```python
from build123d import *

# Parameters (mm, degrees)
EXTRUDE_1_DEPTH      = 6
SKETCH_2_W           = 10
SKETCH_2_H           = 5
CUT_EXTRUDE_1_DEPTH  = 31.822070015
SKETCH_3_R           = 1.5
CUT_EXTRUDE_2_DEPTH  = 39.013155617
SKETCH_4_W           = 20
SKETCH_4_H           = 34
CUT_EXTRUDE_3_DEPTH  = 2
SKETCH_5_R           = 1.25
CUT_EXTRUDE_4_DEPTH  = 31.495901364
FILLET_2_R           = 1.5
SKETCH_9_W           = 1.5
SKETCH_9_H           = 35
CUT_EXTRUDE_10_DEPTH = 31.822070015
SKETCH_10_W          = 2
SKETCH_10_H          = 6
EXTRUDE_2_DEPTH      = 6
SKETCH_11_R          = 1.25
CUT_EXTRUDE_11_DEPTH = 30.618406439


with BuildPart() as part:
    # 草图1 → 凸台-拉伸1 (new body)
    with BuildSketch(Plane.XY):
        Polygon((-25, -17), (-25, 17), (-22, 17), (-22, 11), (-12, 11), (-12, 17), (12, 17), (12, 11), (22, 11), (22, 17), (25, 17), (25, -17), (22, -17), (22, -11), (12, -11), (12, -17), (-12, -17), (-12, -11), (-22, -11), (-22, -17), align=None)
    extrude(amount=EXTRUDE_1_DEPTH)

    # 草图2 → 切除-拉伸1 (cut, through all)
    with BuildSketch(Plane.XY.offset(6)):
        with Locations((-16, 5)):
            Rectangle(SKETCH_2_W, SKETCH_2_H)
        with Locations((-16, -5)):
            Rectangle(SKETCH_2_W, SKETCH_2_H)
        with Locations((16, -5)):
            Rectangle(SKETCH_2_W, SKETCH_2_H)
        with Locations((16, 5)):
            Rectangle(SKETCH_2_W, SKETCH_2_H)
    extrude(amount=-CUT_EXTRUDE_1_DEPTH, mode=Mode.SUBTRACT)

    # 草图3 → 切除-拉伸2 (cut, through all)
    with BuildSketch(Plane.XZ.offset(11)):
        with Locations(Location((-16, 3, 0), (0, 0, 270))):
            Circle(SKETCH_3_R)
        with Locations(Location((16, 3, 0), (0, 0, 270))):
            Circle(SKETCH_3_R)
    extrude(amount=-CUT_EXTRUDE_2_DEPTH, mode=Mode.SUBTRACT)

    # 草图4 → 切除-拉伸3 (cut)
    with BuildSketch(Plane.XY.offset(6)):
        Rectangle(SKETCH_4_W, SKETCH_4_H)
    extrude(amount=-CUT_EXTRUDE_3_DEPTH, mode=Mode.SUBTRACT)

    # 草图5 → 切除-拉伸4 (cut, through all)
    with BuildSketch(Plane.XY.offset(4)):
        with Locations((-6, 6)):
            Circle(SKETCH_5_R)
        with Locations((6, 6)):
            Circle(SKETCH_5_R)
        with Locations((-6, -6)):
            Circle(SKETCH_5_R)
        with Locations((6, -6)):
            Circle(SKETCH_5_R)
    extrude(amount=-CUT_EXTRUDE_4_DEPTH, mode=Mode.SUBTRACT)

    # 圆角2
    fillet_2_edges = [part.edges().sort_by_distance(p)[0] for p in [
        (-11, 7.5, 3),
        (-11, 2.5, 3),
        (-21, 2.5, 3),
        (-21, 7.5, 3),
        (-21, -7.5, 3),
        (-21, -2.5, 3),
        (-11, -2.5, 3),
        (-11, -7.5, 3),
        (21, -2.5, 3),
        (21, -7.5, 3),
        (11, -7.5, 3),
        (11, -2.5, 3),
        (21, 7.5, 3),
        (21, 2.5, 3),
        (11, 2.5, 3),
        (11, 7.5, 3),
    ]]
    fillet(fillet_2_edges, radius=FILLET_2_R)

    # 草图9 → 切除-拉伸10 (cut, through all)
    with BuildSketch(Plane.XY.offset(6)):
        with Locations((-24.25, -0.5)):
            Rectangle(SKETCH_9_W, SKETCH_9_H)
        with Locations((24.25, -0.5)):
            Rectangle(SKETCH_9_W, SKETCH_9_H)
    extrude(amount=-CUT_EXTRUDE_10_DEPTH, mode=Mode.SUBTRACT)

    # 草图10 → 凸台-拉伸2 (add)
    with BuildSketch(Plane.XY.offset(6)):
        with Locations((-21, 14)):
            Rectangle(SKETCH_10_W, SKETCH_10_H)
        with Locations((21, 14)):
            Rectangle(SKETCH_10_W, SKETCH_10_H)
        with Locations((21, -14)):
            Rectangle(SKETCH_10_W, SKETCH_10_H)
        with Locations((-21, -14)):
            Rectangle(SKETCH_10_W, SKETCH_10_H)
    extrude(amount=-EXTRUDE_2_DEPTH)

    # 草图11 → 切除-拉伸11 (cut, through all)
    with BuildSketch(Plane.XY.offset(6)):
        with Locations((-19.2, 11.8)):
            Circle(SKETCH_11_R)
        with Locations((-12.8, 11.8)):
            Circle(SKETCH_11_R)
        with Locations((12.8, 11.8)):
            Circle(SKETCH_11_R)
        with Locations((19.2, 11.8)):
            Circle(SKETCH_11_R)
        with Locations((19.2, -11.8)):
            Circle(SKETCH_11_R)
        with Locations((12.8, -11.8)):
            Circle(SKETCH_11_R)
        with Locations((-12.8, -11.8)):
            Circle(SKETCH_11_R)
        with Locations((-19.2, -11.8)):
            Circle(SKETCH_11_R)
    extrude(amount=-CUT_EXTRUDE_11_DEPTH, mode=Mode.SUBTRACT)


solid = part.part
```
Part model, mm, in its own coordinate system. A direction names the side the tool comes from. Give positions to 0.01 mm unless a question says otherwise; leave off trailing zeros. Order: outer loops, then holes, each group sorted by start corner. A loop starts at its lowest first (then second) coordinate and runs counter-clockwise, first axis right, second up. Notation, with made-up numbers: M -26,66.5 L 4,66.5 A36 cw 4,105.5 Z; hole C 8.5,0 d10. An arc over 180 degrees is marked long. Use a Markdown table: item, result. Add a question column.
(1) Saw through at C-C, the plane x = 6. Give the cut face in (y, z), and give its area (3 significant figures).
(2) 3-axis set-ups, long thin cutter, end or side, ignore diameter. For faces 1 (the face through (-20.57, -7.05, 2.96)), 2 (the face through (-15.55, -0.04, 1.57)), 3 (the face through (-20, -15, 3)): which of +Z, -Z, +X, -X, +Y, -Y reach the whole face in a straight line?
(3) Saw through at D-D, the plane y = 1. Give the cut face in (x, z).
(4) Mould opens along Y. For faces 4 (the face through (-12, 15, 3)), 5 (the face through (0, -17, 2)), 6 (the face through (11.896, 10.937, 3.042)) say: +Y half, -Y half, draft (parallel to the pull), parting line (faces both ways), or undercut.
(5) Saw through at B-B, the plane y = -11.8. Give the cut face in (x, z).
(6) Saw through at A-A, the plane x = 16. Give the cut face in (y, z), and give its area (3 significant figures).
(7) Probe line 1 along Y through (x, z) = (6, 2.75); line 2 along X through (y, z) = (10.2, 3); line 3 along X through (y, z) = (11.8, 1.8). List the from-to ranges inside material, lowest first. Write a range as [from, to].
(8) Drop flat-ended pins along their axis: P1, Ø2.5, axis at x = -16, z = 3, coming from the -Y side; P2, Ø1.8, axis at x = 15, z = 4, coming from the +Y side; P3, Ø4, axis at x = -12.8, y = -11.8, coming from the -Z side; P4, Ø12, axis at x = 2, y = -10.5, coming from the +Z side. Give the stop position or say it passes through.
Answer key:
| question | item | result |
|---|---|---|
| 1 | outline | M -17,0 L -7.25,0 L -7.25,4 L -17,4 Z; M -4.75,0 L 4.75,0 L 4.75,4 L -4.75,4 Z; M 7.25,0 L 17,0 L 17,4 L 7.25,4 Z |
| 1 | area | 116 mm^2 |
| 2 | face 1 | +Z, -Z |
| 2 | face 2 | +Y, -Y |
| 2 | face 3 | +Z, -Z, -Y |
| 3 | outline | M -23.5,0 L 23.5,0 L 23.5,6 L 10,6 L 10,4 L -10,4 L -10,6 L -23.5,6 Z; hole C -16,3 d3; hole C 16,3 d3 |
| 4 | face 4 | draft |
| 4 | face 5 | -Y half |
| 4 | face 6 | undercut |
| 5 | outline | M -23.5,0 L -20.45,0 L -20.45,6 L -23.5,6 Z; M -11.55,0 L 11.55,0 L 11.55,6 L 10,6 L 10,4 L -10,4 L -10,6 L -11.55,6 Z; M 20.45,0 L 23.5,0 L 23.5,6 L 20.45,6 Z |
| 6 | outline | M -11,0 L -7.5,0 L -7.5,1.5 L -11,1.5 Z; M -11,4.5 L -7.5,4.5 L -7.5,6 L -11,6 Z; M -2.5,0 L 2.5,0 L 2.5,1.5 L -2.5,1.5 Z; M -2.5,4.5 L 2.5,4.5 L 2.5,6 L -2.5,6 Z; M 7.5,0 L 11,0 L 11,1.5 L 7.5,1.5 Z; M 7.5,4.5 L 11,4.5 L 11,6 L 7.5,6 Z |
| 6 | area | 36.0 mm^2 |
| 7 | line 1 | [-17, -7.25], [-4.75, 4.75], [7.25, 17] |
| 7 | line 2 | [-23.5, -17.5], [-14.5, 14.5], [17.5, 23.5] |
| 7 | line 3 | [-23.5, -20.45], [-11.55, 11.55], [20.45, 23.5] |
| 8 | P1 | through |
| 8 | P2 | y = 11 |
| 8 | P3 | z = 0 |
| 8 | P4 | z = 4 |
